from build123d import *

# Parameters (mm, degrees)
SKETCH007_R          = 0.5
PAD001_DEPTH         = 1.5
POCKET_DEPTH         = 1.501
POCKET_DEPTH_BACK    = 0.001
SKETCH_R             = 0.8
SKETCH_R_2           = 2.7
POCKET001_DEPTH      = 1.501
POCKET001_DEPTH_BACK = 0.001


with BuildPart() as part:
    # Sketch007 → Pad001 (new body)
    with BuildSketch(Plane.XY):
        with BuildLine():
            Line((-20, 0), (-20, -0.292893))
            ThreePointArc((-20.707107, -1), (-20, -1), (-20, -0.292893))
            Line((-20.707107, -1), (-21.5, -1))
            ThreePointArc((-21.5, -1), (-22.25, -1.75), (-21.5, -2.5))
            Line((-21.5, -2.5), (-18.063508, -2.5))
            ThreePointArc((-18.063508, -2.5), (-17.420322, -1.829006), (-17, -1))
            Line((-17, 0), (-17, -1))
            ThreePointArc((-16, 0), (-16.5, 0.5), (-17, 0))
            Line((-16, 0), (-15.5, 0))
            ThreePointArc((-4.98789, 1.828965), (-10.284682, 1.148622), (-15.5, 0))
            ThreePointArc((-3, 0), (-3.592665, 1.350631), (-4.98789, 1.828965))
            Line((-2.5, 0), (-3, 0))
            ThreePointArc((-1.5, 0), (-2, 0.5), (-2.5, 0))
            Line((-1.5, -1.5), (-1.5, 0))
            ThreePointArc((-1.5, -1.5), (0, -2.5), (1.5, -1.5))
            Line((1.5, 0), (1.5, -1.5))
            ThreePointArc((2.5, 0), (2, 0.5), (1.5, 0))
            Line((2.5, 0), (3, 0))
            ThreePointArc((4.98789, 1.828965), (3.592665, 1.350631), (3, 0))
            ThreePointArc((15.5, 0), (10.284682, 1.148622), (4.98789, 1.828965))
            Line((16, 0), (15.5, 0))
            ThreePointArc((17, 0), (16.5, 0.5), (16, 0))
            Line((17, 0), (17, -1.5))
            ThreePointArc((17, -1.5), (18.5, -2.5), (20, -1.5))
            Line((20, -1.5), (20, 0))
            Line((20, 0), (20.436997, 3.505138))
            ThreePointArc((20.436997, 3.505138), (19.396762, 6.724105), (16.261564, 7.994684))
            ThreePointArc((14.353635, 10.853725), (14.494893, 8.88186), (16.261564, 7.994684))
            ThreePointArc((14.353635, 10.853725), (14.268742, 12.300184), (13, 13))
            Line((13, 13), (9, 13))
            ThreePointArc((9, 13), (7.6704, 12.194379), (7.769004, 10.642884))
            ThreePointArc((7.097708, 7.751052), (8.075873, 9.047817), (7.769004, 10.642884))
            Line((3.061388, 5.512462), (7.097708, 7.751052))
            ThreePointArc((1.717585, 5.874647), (2.316142, 5.421425), (3.061388, 5.512462))
            ThreePointArc((1.717585, 5.874647), (0, 6.85), (-1.717585, 5.874647))
            ThreePointArc((-3.061388, 5.512462), (-2.316142, 5.421425), (-1.717585, 5.874647))
            Line((-7.097708, 7.751052), (-3.061388, 5.512462))
            ThreePointArc((-7.769004, 10.642884), (-8.075873, 9.047817), (-7.097708, 7.751052))
            ThreePointArc((-7.769004, 10.642884), (-7.6704, 12.19438), (-9, 13))
            Line((-13, 13), (-9, 13))
            ThreePointArc((-13, 13), (-14.268742, 12.300184), (-14.353635, 10.853725))
            ThreePointArc((-16.261564, 7.994684), (-14.494893, 8.88186), (-14.353635, 10.853725))
            ThreePointArc((-16.261564, 7.994684), (-19.396762, 6.724105), (-20.436997, 3.505138))
            Line((-20, 0), (-20.436997, 3.505138))
        make_face()
        with Locations((18.5, -1.5)):
            Circle(SKETCH007_R, mode=Mode.SUBTRACT)
        with Locations((0, -1.5)):
            Circle(SKETCH007_R, mode=Mode.SUBTRACT)
    extrude(amount=PAD001_DEPTH)

    # Sketch006 → Pocket (cut, two sides)
    with BuildSketch(Plane.XY) as pocket_sk:
        with BuildLine():
            ThreePointArc((-13, 12), (-13.5, 11.5), (-13, 11))
            Line((-13, 11), (-9, 11))
            ThreePointArc((-9, 11), (-8.5, 11.5), (-9, 12))
            Line((-13, 12), (-9, 12))
        make_face()
        with BuildLine():
            ThreePointArc((9, 12), (8.5, 11.5), (9, 11))
            Line((9, 11), (13, 11))
            ThreePointArc((13, 11), (13.5, 11.5), (13, 12))
            Line((9, 12), (13, 12))
        make_face()
    extrude(amount=POCKET_DEPTH, mode=Mode.SUBTRACT)
    extrude(pocket_sk.sketch, amount=-POCKET_DEPTH_BACK, mode=Mode.SUBTRACT)

    # Sketch → Pocket001 (cut, two sides)
    with BuildSketch(Plane.XY) as pocket001_sk:
        with Locations((-9.083242, 4.85)):
            Circle(SKETCH_R)
        with Locations((9.083242, 4.85)):
            Circle(SKETCH_R)
        with Locations((0, 4.85)):
            Circle(SKETCH_R)
        with Locations((-16.467726, 4)):
            Circle(SKETCH_R_2)
        with Locations((16.467726, 4)):
            Circle(SKETCH_R_2)
    extrude(amount=POCKET001_DEPTH, mode=Mode.SUBTRACT)
    extrude(pocket001_sk.sketch, amount=-POCKET001_DEPTH_BACK, mode=Mode.SUBTRACT)


solid = part.part
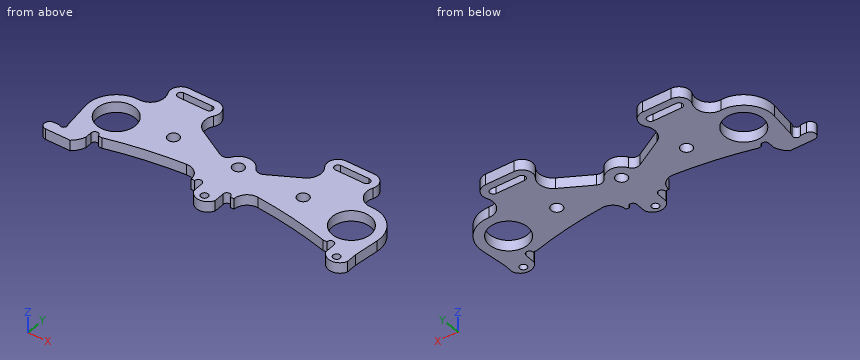
Model file for the job. Use its own axes, mm. Round coordinates to 2 decimals unless told otherwise and drop trailing zeros. Loops run counter-clockwise (first coordinate to the right, second up) from the corner with the lowest first, then second, coordinate; pieces in that order, holes last. Notation, with made-up numbers: (-24.5, 49) -> (21.5, 49) arc R6 ccw to (21.5, 53) -> close; hole circle Ø7 at (70.5, -21.5). An arc over 180 degrees is marked (long way). Answer as CSV lines item,"result". Start each with the question number.
1) Slice it at B-B (y = 11.5). List the corners of the cut face in (x, z).
2) Slice it at D-D (y = 4.85). List the corners of the cut face in (x, z), plus the area to 3 significant figures.
3) Slice it at A-A (x = 0). List the corners of the cut face in (y, z), plus the area to 3 significant figures.
4) Probe line 1 along Y through (x, z) = (0, 1); line 2 along X through (y, z) = (3, 0.6); line 3 along X through (y, z) = (5, 0.4). List the from-to ranges inside material, lowest first.
5) Pin check, flat tips, straight feed: P1, Ø4.5, axis at x = 16.47, y = 4, coming from the -Z side; P2, Ø0.6, axis at x = -15.5, z = 0.5, coming from the -Y side. Stop position of each tip, or through.
6) Slice it at C-C (x = -12.5). List the corners of the cut face in (y, z).
Filled in:
1,outline,"(-14.5, 0) -> (-13.5, 0) -> (-13.5, 1.5) -> (-14.5, 1.5) -> close; (-8.5, 0) -> (-7.5, 0) -> (-7.5, 1.5) -> (-8.5, 1.5) -> close; (7.5, 0) -> (8.5, 0) -> (8.5, 1.5) -> (7.5, 1.5) -> close; (13.5, 0) -> (14.5, 0) -> (14.5, 1.5) -> (13.5, 1.5) -> close"
2,outline,"(-20.38, 0) -> (-19.03, 0) -> (-19.03, 1.5) -> (-20.38, 1.5) -> close; (-13.91, 0) -> (-9.88, 0) -> (-9.88, 1.5) -> (-13.91, 1.5) -> close; (-8.28, 0) -> (-0.8, 0) -> (-0.8, 1.5) -> (-8.28, 1.5) -> close; (0.8, 0) -> (8.28, 0) -> (8.28, 1.5) -> (0.8, 1.5) -> close; (9.88, 0) -> (13.91, 0) -> (13.91, 1.5) -> (9.88, 1.5) -> close; (19.03, 0) -> (20.38, 0) -> (20.38, 1.5) -> (19.03, 1.5) -> close"
2,area,"38.6 mm2"
3,outline,"(-2.5, 0) -> (-2, 0) -> (-2, 1.5) -> (-2.5, 1.5) -> close; (-1, 0) -> (4.05, 0) -> (4.05, 1.5) -> (-1, 1.5) -> close; (5.65, 0) -> (6.85, 0) -> (6.85, 1.5) -> (5.65, 1.5) -> close"
3,area,"10.1 mm2"
4,line 1,"y = -2.5 to -2, -1 to 4.05, 5.65 to 6.85"
4,line 2,"x = -20.37 to -18.98, -13.96 to 13.96, 18.98 to 20.37"
4,line 3,"x = -20.34 to -18.98, -13.96 to -9.87, -8.3 to -0.79, 0.79 to 8.3, 9.87 to 13.96, 18.98 to 20.34"
5,P1,"passes through"
5,P2,"stops at y = 0"
6,outline,"(0.72, 0) -> (11, 0) -> (11, 1.5) -> (0.72, 1.5) -> close; (12, 0) -> (13, 0) -> (13, 1.5) -> (12, 1.5) -> close"
